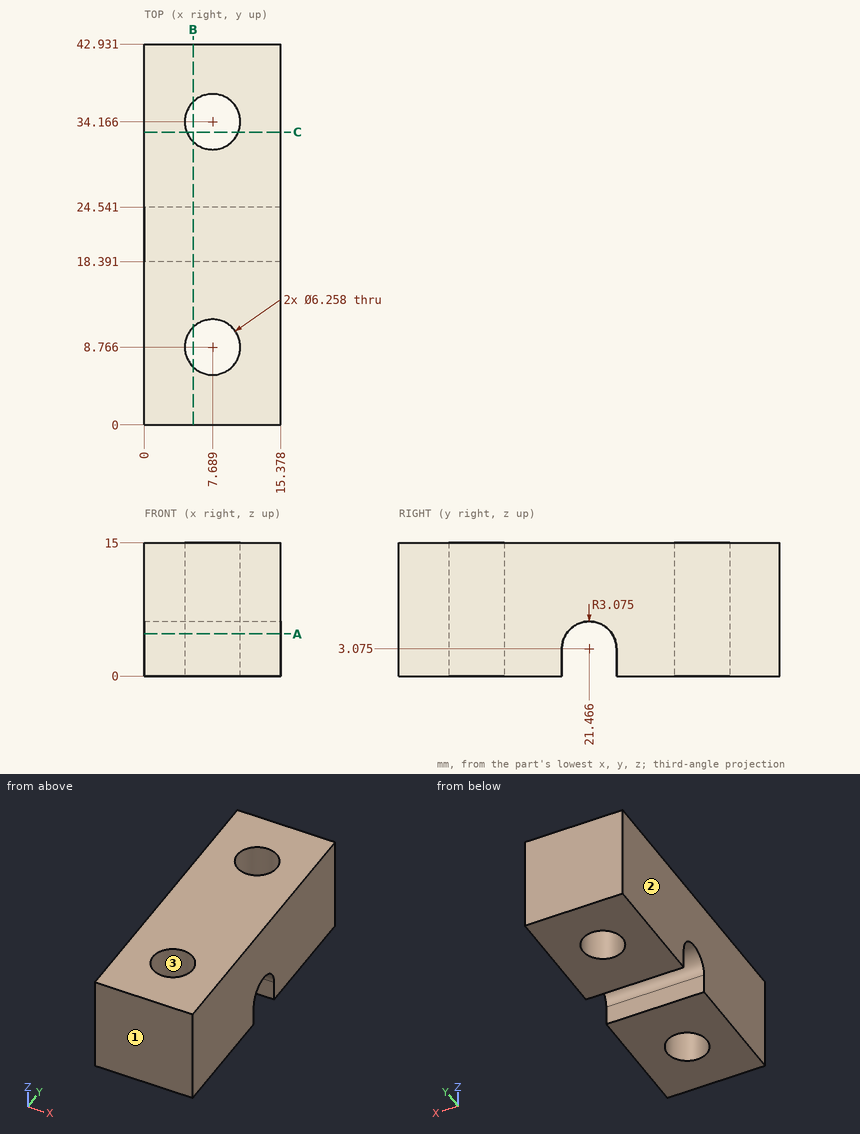
Study the drawing (mm; zero at the part's minimum x, y, z) and answer. Round coordinates to 2 decimals unless told otherwise and drop trailing zeros. Write each loop counter-clockwise with the first axis right and the second up, starting at its lowest first coordinate (ties: lowest second). Pieces come first, ordered by that corner, then holes.
1) A cutting plane is placed at B-B on x = 5.5. Give the number of separate pieces and of enclosed holes in the cut face, and give its area (3 significant figures).
2) A flat-ended cylindrical pin translates along its axis: P1, Ø4, axis at x = 7.69, y = 34.17, coming from the -Z side. Find the tip coordinate at first contact, or state that the pin passes through.
3) A cutting plane is placed at C-C on y = 33. Determine the outline of the cut face in (x, z) (1 decimal).
4) Determine the mould class of the marked faces 1, 2 and 3 for opening direction Y: pulls with the +Y half, pulls with the -Y half, needs draft (parallel to the pull), parting line crosses it, or undercut.
5) Consider probe 1 along Y at (x, z) = (11.5, 3); probe 2 along Y at (x, z) = (8, 7); probe 3 along Y at (x, z) = (5.5, 11.5). Determine where each line is inside the solid, lowest interval first.
6) A cutting plane is placed at A-A on z = 4.75. Determine the outline of the cut face in (x, y) (1 decimal).
Entries:
1. separate pieces: 3
1. enclosed holes: 0
1. area: 476 mm2
2. P1: passes through
3. outline: (0, 0) - (4.8, 0) - (4.8, 15) - (0, 15) - close; (10.6, 0) - (15.4, 0) - (15.4, 15) - (10.6, 15) - close
4. face 1: pulls with the -Y half
4. face 2: needs draft
4. face 3: undercut
5. probe 1: y = 0 to 18.39, 24.54 to 42.93
5. probe 2: y = 0 to 5.65, 11.88 to 31.05, 37.28 to 42.93
5. probe 3: y = 0 to 6.53, 11 to 31.93, 36.4 to 42.93
6. outline: (0, 0) - (15.4, 0) - (15.4, 18.9) - (0, 18.9) - close; (0, 24) - (15.4, 24) - (15.4, 42.9) - (0, 42.9) - close; hole circle Ø6.3 at (7.7, 8.8); hole circle Ø6.3 at (7.7, 34.2)
